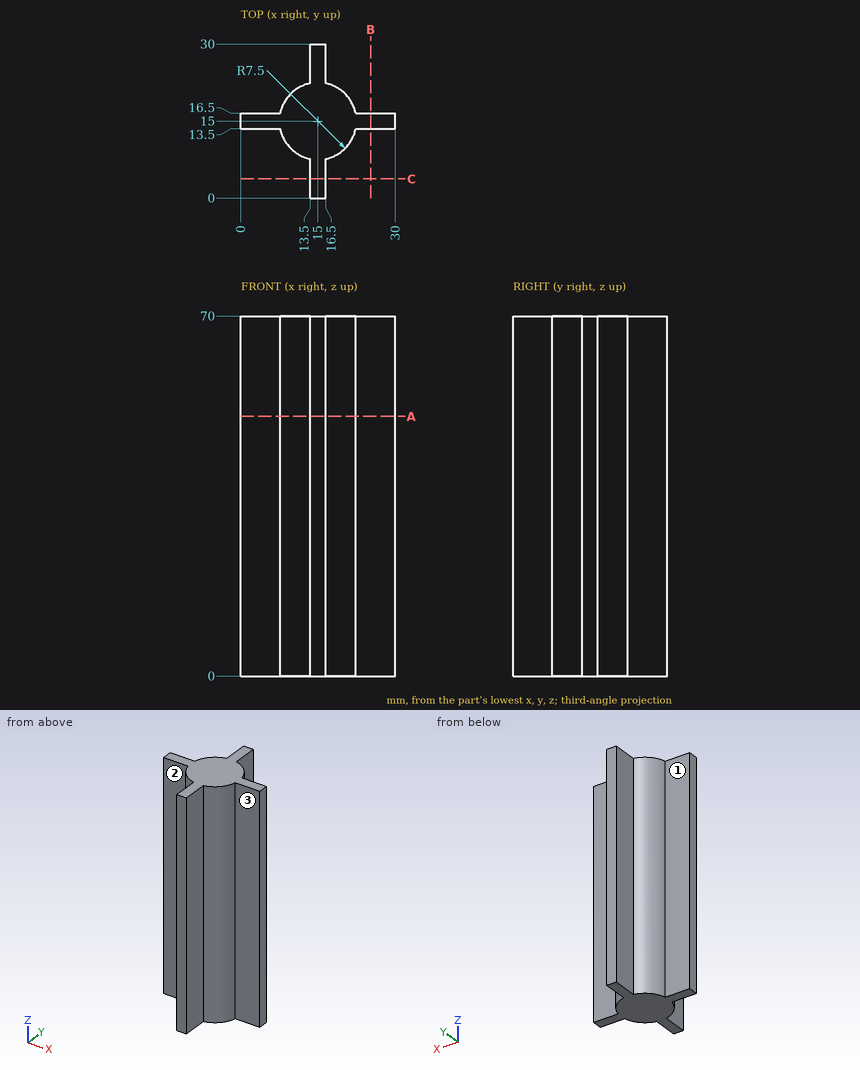
Geometry: see drawing. Coordinates: mm, zero at the bounding-box minimum. A direction names the side the tool comes from. Round coordinates to 2 decimals unless told otherwise and drop trailing zeros. Write each loop counter-clockwise with the first axis right and the second up, starting at its lowest first coordinate (ties: lowest second). Pieces come first, ordered by that corner, then holes. Notation, with made-up numbers: (42.5, 38) - (100.5, 38) arc R14 cw to (100.5, 46) - close; hole circle Ø2 at (50.25, 89.25). An arc over 180 degrees is marked (long way). Use CSV: the item, a comma, the result in double quotes. Start each with the question number.
(1) Cut plane B-B, the plane x = 25.25. Return loops of the section in (y, z), and give its area (3 significant figures).
(2) Cut plane A-A, the plane z = 50.5. Return loops of the section in (x, y), and give its area (3 significant figures).
(3) Material intervals for probe 1 along Y at (x, z) = (2.75, 26.5); probe 2 along X at (y, z) = (12, 10.5), sorted ascending. Write a range as [from, to].
(4) Set-up query: the marked faces 1, 2 and 3. Return all of +Z, -Z, +X, -X, +Y, -Y with unobstructed straight access to the full face (end or side cutting, diameter ignored); none if empty.
(5) First-contact query: pin 1 Ø8.5 at (x, z) = (27.5, 36) entering from -Y; pin 2 Ø4 at (y, z) = (3.5, 11.5) entering from -X; pin 3 Ø8.5 at (x, z) = (4.5, 23.5) entering from -Y. Flat tips, straight axial feed; report the tip coordinate or a pass-through.
Geometry says:
1,outline,"(13.5, 0) - (16.5, 0) - (16.5, 70) - (13.5, 70) - close"
1,area,"210 mm²"
2,outline,"(0, 13.5) - (7.65, 13.5) arc R7.5 ccw to (13.5, 7.65) - (13.5, 0) - (16.5, 0) - (16.5, 7.65) arc R7.5 ccw to (22.35, 13.5) - (30, 13.5) - (30, 16.5) - (22.35, 16.5) arc R7.5 ccw to (16.5, 22.35) - (16.5, 30) - (13.5, 30) - (13.5, 22.35) arc R7.5 ccw to (7.65, 16.5) - (0, 16.5) - close"
2,area,"267 mm²"
3,probe 1,"[13.5, 16.5]"
3,probe 2,"[8.13, 21.87]"
4,face 1,"+Z, -Z, -X, +Y"
4,face 2,"+Z, -Z, -X, -Y"
4,face 3,"+Z, -Z, +X, -Y"
5,pin 1,"y = 13.5"
5,pin 2,"x = 13.5"
5,pin 3,"y = 10.85"
